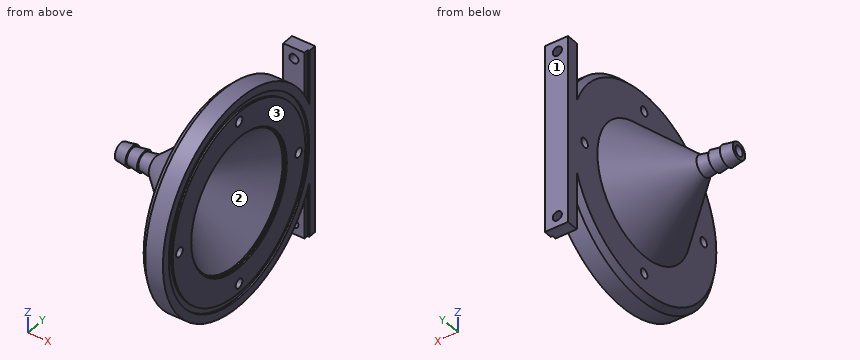
from build123d import *

# Parameters (mm, degrees)
M3_CLEARANCE_HOLE1_D     = 3.4
M3_CLEARANCE_HOLE1_DEPTH = 8.566
M3_CLEARANCE_HOLE1_TIP   = 1.021463052
CHAMFER1_SIZE            = 2
BOSS_EXTRUDE1_DEPTH      = 35
SKETCH9_R                = 1.7
CUT_EXTRUDE1_DEPTH       = 10


with BuildPart() as part:
    # Sketch1 → Revolve17 (revolve)
    with BuildSketch(Plane.XY, mode=Mode.PRIVATE) as revolve17_sk:
        Polygon((16.809150592, 39), (16.809150592, 34.5), (24.708150592, 34.5), (24.708150592, 36), (25.375150592, 36), (25.375150592, 39), align=None)
        Polygon((-14.010170791, 3.15), (-14.010170791, 3.8), (-18.343504124, 3.15), (-18.343504124, 1.9), (0, 1.9), (24.243150592, 23.934), (24.809150592, 23.934), (24.809150592, 24.5), (25.375150592, 24.5), (25.375150592, 34), (24.708150592, 34), (24.708150592, 34.5), (16.809150592, 34.5), (16.809150592, 23.934), (-5.343504124, 3.8), (-9.676837458, 3.15), (-9.676837458, 3.8), align=None)
    revolve(revolve17_sk.sketch.rotate(Axis((-801.927103621, 0, 0), (1, 0, 0)), 90), axis=Axis((-801.927103621, 0, 0), (1, 0, 0)))

    # M3 Clearance Hole1
    with Locations(Plane.ZY.offset(-16.809150592)):
        with Locations((0, -30.5), (0, 30.5), (30.5, 0), (-30.5, 0)):
            Hole(M3_CLEARANCE_HOLE1_D / 2, depth=M3_CLEARANCE_HOLE1_DEPTH)
            with Locations((0, 0, -(M3_CLEARANCE_HOLE1_DEPTH + M3_CLEARANCE_HOLE1_TIP / 2))):  # 118° drill point
                Cone(0, M3_CLEARANCE_HOLE1_D / 2, M3_CLEARANCE_HOLE1_TIP, mode=Mode.SUBTRACT)

    # Chamfer1
    chamfer1_edges = [part.edges().sort_by_distance(p)[0] for p in [
        (16.809150592, 0, -39),
    ]]
    chamfer(chamfer1_edges, length=CHAMFER1_SIZE)

    # Sketch1_11 → Boss-Extrude1 (add, symmetric)
    with BuildSketch(Plane.XY):
        Polygon((16.809150592, 39), (16.809150592, 34.5), (24.708150592, 34.5), (24.708150592, 36), (25.375150592, 36), (25.375150592, 39), align=None)
    extrude(amount=BOSS_EXTRUDE1_DEPTH, both=True)

    # Sketch9 → Cut-Extrude1 (cut)
    with BuildSketch(Plane(origin=(0, 34.5, 0), x_dir=(-1, 0, 0), z_dir=(0, -1, 0))):
        with Locations(Location((-20.758650592, -31, 0), (0, 0, 90))):
            Circle(SKETCH9_R)
        with Locations((-20.758650592, 31)):
            Circle(SKETCH9_R)
    extrude(amount=-CUT_EXTRUDE1_DEPTH, mode=Mode.SUBTRACT)


solid = part.part
The listing builds one solid part. Answer for the finished solid, in the listing's coordinates (mm). Face numbers are marked on the shaded views. Round coordinates to 2 decimals unless told otherwise and drop trailing zeros. Write each loop counter-clockwise with the first axis right and the second up, starting at its lowest first coordinate (ties: lowest second). Pieces come first, ordered by that corner, then holes. Notation, with made-up numbers: (-32, 60) - (9, 60) arc R30 cw to (9, 82) - close; hole circle Ø3 at (13.5, 87). An arc over 180 degrees is marked (long way). Use a Markdown table: item, result. Add a question column.
1. Consider line 1 (X direction, y = 35.4, z = -31); line 2 (Y direction, x = 23.5, z = 0); line 3 (Y direction, x = 21, z = 0). Determine where each line is inside the solid, lowest interval first.
2. For a pull along Y with two mould halves and no side action, classify the marked faces 1, 2 and 3 as +Y half, -Y half, draft (parallel to the pull), parting line (faces both ways), or undercut.
3. The part is cut by section C-C (x = -1.5). Write down the section's boundary in (y, z).
4. The part is cut by section A-A (z = 0). Give the number of separate pieces and of enclosed holes in the cut face, and give its area (3 significant figures).
5. Flat-ended cylindrical pins translate along their axes: P1, Ø5, axis at x = 8.5, z = 5.5, coming from the +Y side; P2, Ø2.5, axis at y = 30.5, z = 0, coming from the -X side; P3, Ø12, axis at x = 4.5, z = -13, coming from the -Y side; P4, Ø0.5, axis at x = 25, z = -24, coming from the -Y side. Find the tip coordinate at first contact, or state that the pin passes through.
Reported:
| question | item | result |
|---|---|---|
| 1 | line 1 | 16.81 to 19.06, 22.46 to 24.71 |
| 1 | line 2 | -39 to -32.2, -28.8 to -23.26, 23.26 to 28.8, 32.2 to 39 |
| 1 | line 3 | -39 to -32.2, -28.8 to -20.99, 20.99 to 28.8, 32.2 to 39 |
| 2 | face 1 | +Y half |
| 2 | face 2 | undercut |
| 2 | face 3 | draft |
| 3 | outline | circle Ø14.59 at (0, 0); hole circle Ø3.8 at (0, 0) |
| 4 | separate pieces | 4 |
| 4 | enclosed holes | 0 |
| 4 | area | 559 mm^2 |
| 5 | P1 | y = 17.93 |
| 5 | P2 | through |
| 5 | P3 | y = -14.33 |
| 5 | P4 | y = -30.93 |
